CAD build for the part. Positions are in the model's coordinates, mm. Face numbers are marked on the shaded views. Round coordinates to 2 decimals unless told otherwise and drop trailing zeros. Loops run counter-clockwise (first coordinate to the right, second up) from the corner with the lowest first, then second, coordinate; pieces in that order, holes last. Notation, with made-up numbers: (9, 42.5) -> (22, 42.5) arc R27 cw to (22, 59.5) -> close; hole circle Ø1 at (-32.5, 24). An arc over 180 degrees is marked (long way). Answer as CSV lines item,"result".
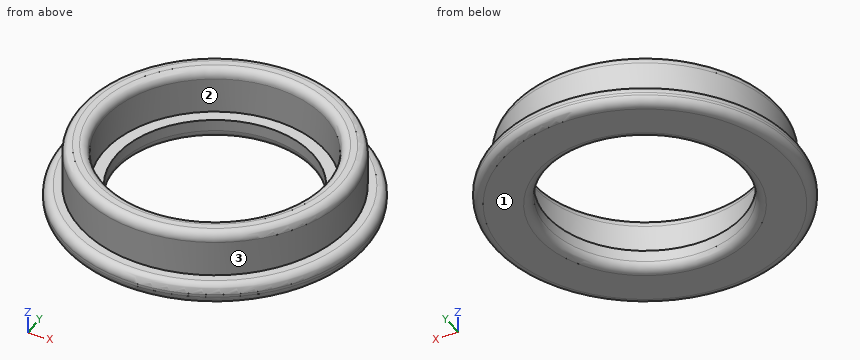
```python
from build123d import *

# Parameters (mm, degrees)
F0_R     = 17
F0_R_2   = 11
F1_DEPTH = 2.3
F2_R     = 15.1
F2_R_2   = 12.4
F3_DEPTH = 5
F4_R     = 1


with BuildPart() as f1:
    # F0 (on Top) → F1 (new body)
    with BuildSketch(Plane.XY):
        Circle(F0_R)
        Circle(F0_R_2, mode=Mode.SUBTRACT)
    extrude(amount=F1_DEPTH)

    # F2 (on face) → F3 (join)
    with BuildSketch(Plane.XY.offset(2.3)):
        Circle(F2_R)
        Circle(F2_R_2, mode=Mode.SUBTRACT)
    extrude(amount=F3_DEPTH)

    # F4
    f4_edges = [f1.edges().sort_by_distance(p)[0] for p in [
        (-17, 0, 0),
        (-11, 0, 0),
        (-15.1, 0, 7.3),
        (-12.4, 0, 7.3),
        (-17, 0, 2.3),
    ]]
    fillet(f4_edges, radius=F4_R)


solid = f1.part
```
Q1. Slice it at A-A, the plane y = 0. Give the cut face in (x, z), and give its area (3 significant figures).
Results:
outline,"(-17, 1) arc R1 ccw to (-16, 0) -> (-12, 0) arc R1 ccw to (-11, 1) -> (-11, 2.3) -> (-12.4, 2.3) -> (-12.4, 6.3) arc R1 ccw to (-13.4, 7.3) -> (-14.1, 7.3) arc R1 ccw to (-15.1, 6.3) -> (-15.1, 2.3) -> (-16, 2.3) arc R1 ccw to (-17, 1.3) -> close; (11, 1) arc R1 ccw to (12, 0) -> (16, 0) arc R1 ccw to (17, 1) -> (17, 1.3) arc R1 ccw to (16, 2.3) -> (15.1, 2.3) -> (15.1, 6.3) arc R1 ccw to (14.1, 7.3) -> (13.4, 7.3) arc R1 ccw to (12.4, 6.3) -> (12.4, 2.3) -> (11, 2.3) -> close"
area,"52.5 mm2"
Q2. Two-plate mould, pull along X, no slides. Class the marked faces 1, 2 and 3: pulls with the +X half, pulls with the -X half, needs draft (parallel to the pull), parting line crosses it, or undercut.
Results:
face 1,"needs draft"
face 2,"undercut"
face 3,"parting line crosses it"
Q3. Slice it at C-C, the plane z = 5.25. Give the cut face in (x, y).
Results:
outline,"circle Ø30.2 at (0, 0); hole circle Ø24.8 at (0, 0)"
Q4. Drop flat-ended pins along their axis: pin 1 Ø2 at (x, z) = (12.5, 4.5) entering from -Y; pin 2 Ø8 at (x, y) = (-7, 3) entering from +Z; pin 3 Ø4 at (y, z) = (11.5, 6) entering from -X. Give the stop position or say it passes through.
Results:
pin 1,"y = -9.79"
pin 2,"z = 2.3"
pin 3,"x = -11.74"
Q5. Probe L1, parallel to Y at x = 0, z = 3.9; L2, parallel to Y at x = 9, z = 4.5; L3, parallel to X at y = 10, z = 5. List the from-to ranges inside material, lowest first. Write a range as [from, to].
Results:
L1,"[-15.1, -12.4], [12.4, 15.1]"
L2,"[-12.12, -8.53], [8.53, 12.12]"
L3,"[-11.31, -7.33], [7.33, 11.31]"
